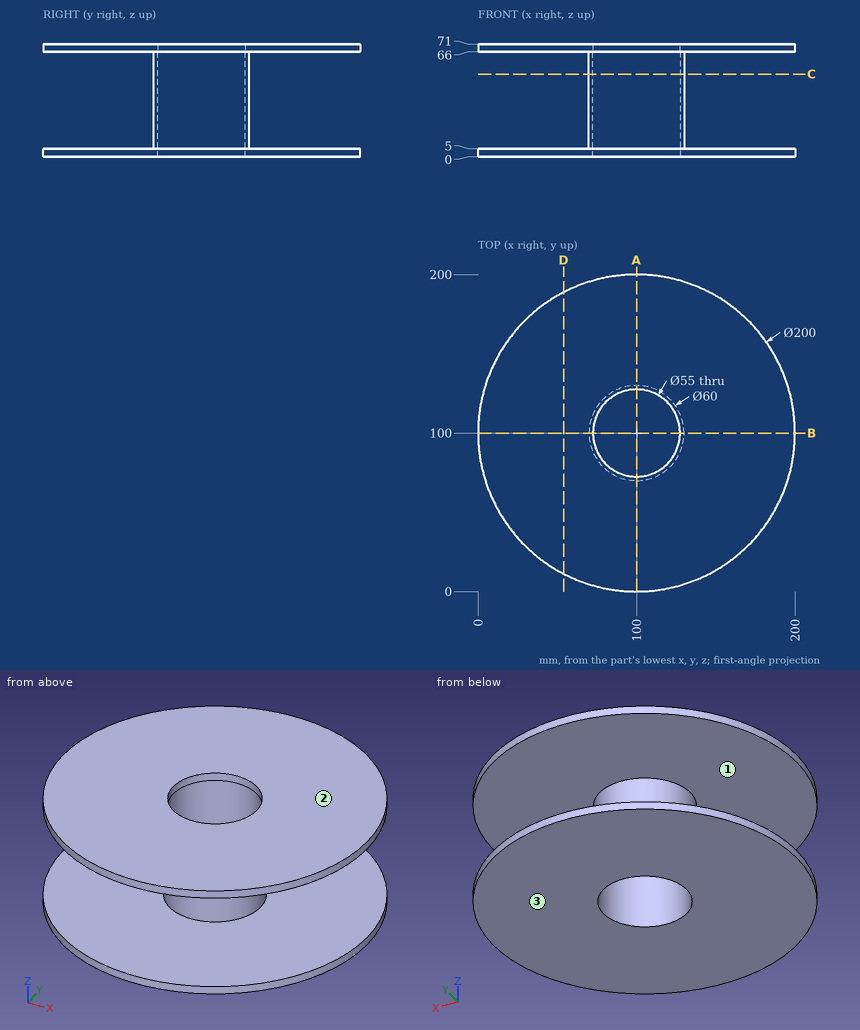
Study the drawing (mm; zero at the part's minimum x, y, z) and answer. Give positions to 0.01 mm unless a question says otherwise; leave off trailing zeros. Order: outer loops, then holes, each group sorted by start corner. A loop starts at its lowest first (then second) coordinate and runs counter-clockwise, first axis right, second up. Notation, with made-up numbers: (82, 38.25) - (123, 38.25) arc R25 ccw to (123, 63.25) - close; hole circle Ø7 at (-10, -6). An arc over 180 degrees is marked (long way). Answer in a Markdown table with one row per item. Add a question column.
Q1. For a pull along Z with two mould halves and no side action, classify the marked faces 1, 2 and 3 as released by +Z, released by -Z, zero draft, split by the parting line, or undercut.
Q2. The part is cut by section A-A (x = 100). Determine the outline of the cut face in (y, z).
Q3. The part is cut by section C-C (z = 52). Determine the outline of the cut face in (x, y), then the cut area to 3 significant figures.
Q4. Find the intervals of material crossed by line 1 along Z through (x, y) = (108, 135.5); line 2 along Y through (x, z) = (100, 68.25); line 3 along X through (y, z) = (102, 36.5), in increasing order. Write a range as [from, to].
Q5. Given P1, Ø12, axis at x = 133, z = 23.5, coming from the -Y side; P2, Ø12, axis at x = 123.5, z = 43.5, coming from the +Y side; P3, Ø2, axis at x = 84, z = 29.5, coming from the +Y side, each flat-ended and moving along its own axis, determine where each tip first touches the part or whether it passes through.
Q6. The part is cut by section D-D (x = 54). Determine the outline of the cut face in (y, z), then the cut area to 3 significant figures.
Determined:
| question | item | result |
|---|---|---|
| 1 | face 1 | undercut |
| 1 | face 2 | released by +Z |
| 1 | face 3 | released by -Z |
| 2 | outline | (0, 0) - (72.5, 0) - (72.5, 71) - (0, 71) - (0, 66) - (70, 66) - (70, 5) - (0, 5) - close; (127.5, 0) - (200, 0) - (200, 5) - (130, 5) - (130, 66) - (200, 66) - (200, 71) - (127.5, 71) - close |
| 3 | outline | circle Ø60 at (100, 100); hole circle Ø55 at (100, 100) |
| 3 | area | 452 mm² |
| 4 | line 1 | z = [0, 5], [66, 71] |
| 4 | line 2 | y = [0, 72.5], [127.5, 200] |
| 4 | line 3 | x = [70.07, 72.57], [127.43, 129.93] |
| 5 | P1 | stops at y = 86.92 |
| 5 | P2 | stops at y = 124.37 |
| 5 | P3 | stops at y = 125.98 |
| 6 | outline | (11.21, 0) - (188.79, 0) - (188.79, 5) - (11.21, 5) - close; (11.21, 66) - (188.79, 66) - (188.79, 71) - (11.21, 71) - close |
| 6 | area | 1,780 mm² |
